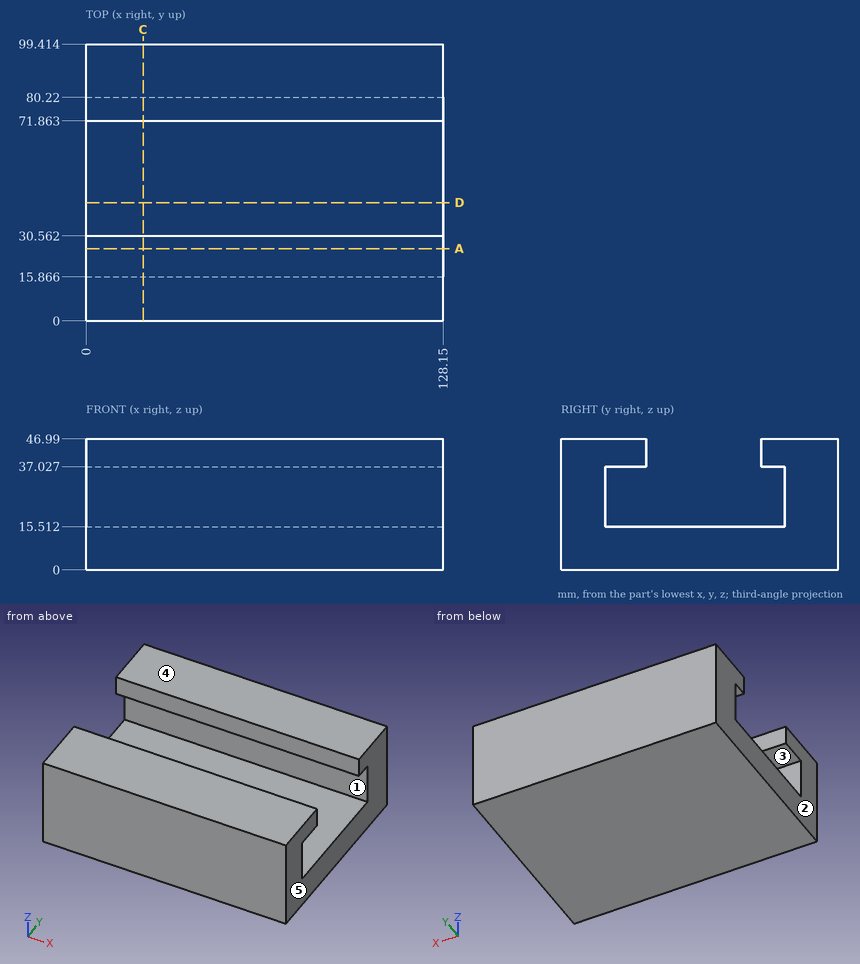
Verification items for this drawing (mm, ordinates from the low corner). A direction names the side the tool comes from. Give positions to 0.01 mm unless a question says otherwise; leave off trailing zeros. Loops run counter-clockwise (first coordinate to the right, second up) from the corner with the lowest first, then second, coordinate; pieces in that order, holes last. Notation, with made-up numbers: M -26,58 L -12,58 A23 cw -12,88 Z; hole C -31,64 d10. An arc over 180 degrees is marked long. Answer as a JSON object with one key per item and string values. Group by question number.
Q1. Material ranges on line 1 along Z through (x, y) = (122.5, 18); line 2 along Y through (x, z) = (33.5, 33) (1 decimal); line 3 along Z through (x, y) = (67, 70.5), recorded low to high. Write a range as [from, to].
Q2. Cross-section at A-A on y = 26. Record the cut outline in (x, z).
Q3. Cross-section at C-C on x = 20.5. Record the cut outline in (y, z) (1 decimal), then the cut area to 3 significant figures.
Q4. Access from +Z, -Z, +X, -X, +Y, -Y to the whole of each face (thin tool, end or side, straight path). Record for the marked faces 1 and 2.
Q5. Release check for a two-part mould opening along Z. For the marked faces 3, 4 and 5 record: released by +Z, released by -Z, zero draft, split by the parting line, or undercut.
Q6. Cross-section at D-D on y = 42.5. Record the cut outline in (x, z).
Evaluation:
{
 "1": {"line 1": "z = [0, 15.51], [37.03, 46.99]", "line 2": "y = [0, 15.9], [80.2, 99.4]", "line 3": "z = [0, 15.51]"},
 "2": {"outline": "M 0,0 L 128.15,0 L 128.15,15.51 L 0,15.51 Z; M 0,37.03 L 128.15,37.03 L 128.15,46.99 L 0,46.99 Z"},
 "3": {"outline": "M 0,0 L 99.4,0 L 99.4,47 L 71.9,47 L 71.9,37 L 80.2,37 L 80.2,15.5 L 15.9,15.5 L 15.9,37 L 30.6,37 L 30.6,47 L 0,47 Z", "area": "2,880 mm2"},
 "4": {"face 1": "+X, -X", "face 2": "+Z, -Z, -X, +Y, -Y"},
 "5": {"face 3": "undercut", "face 4": "released by +Z", "face 5": "zero draft"},
 "6": {"outline": "M 0,0 L 128.15,0 L 128.15,15.51 L 0,15.51 Z"}
}
